Source: CAD feature listing. Evaluate the final solid. Frame: model axes, mm. Give positions to 0.01 mm unless a question says otherwise; leave off trailing zeros. Order: outer loops, then holes, each group sorted by start corner. A loop starts at its lowest first (then second) coordinate and runs counter-clockwise, first axis right, second up.
1) Material intervals for line 1 (Y direction, x = 17.5, z = 1); line 2 (Y direction, x = 7.5, z = 18), sorted ascending.
2) First-contact query: P1, Ø1.8, axis at y = -407.5, z = 10.5, coming from the -X side; P2, Ø12, axis at x = 6.5, z = 17.5, coming from the -Y side; P3, Ø8, axis at y = 407.793, z = 10, coming from the -X side; P4, Ø3.5, axis at y = -407.793, z = 10, coming from the +X side. Flat tips, straight axial feed; report the tip coordinate or a pass-through.
3) Section B-B, the plane x = 7.75. Return loops of the section in (y, z), plus the area to 3 significant figures.
```python
from build123d import *

# Parameters (mm, degrees)
F0_W     = 20
F0_H     = 20
F1_DEPTH = 417.793
F2_SIZE2 = 19.99999
F2_SIZE  = 19.99999
F3_SIZE  = 19.99999
F4_R     = 3
F5_DEPTH = 4
F6_R     = 3
F7_DEPTH = 4


# Not quite as in the source:
# - a fillet or chamfer is up to 0.001 mm smaller than in the source, because OpenCascade refuses the exact size


with BuildPart() as f1:
    # F0 (on Front) → F1 (new body, symmetric)
    with BuildSketch(Plane.XZ):
        with Locations((10, 10)):
            Rectangle(F0_W, F0_H)
    extrude(amount=F1_DEPTH, both=True)

    # F2 (size 20 and 20 in the source; OpenCascade refuses exactly that, so slightly less here)
    f2_edges = [f1.edges().sort_by_distance(p)[0] for p in [
        (20, -417.793, 10),
    ]]
    chamfer(f2_edges, length=F2_SIZE, length2=F2_SIZE2)

    # F3 (size 20 in the source; OpenCascade refuses exactly that, so slightly less here)
    f3_edges = [f1.edges().sort_by_distance(p)[0] for p in [
        (20, 417.793, 10),
    ]]
    chamfer(f3_edges, length=F3_SIZE)

    # F4 (on face) → F5 (cut)
    with BuildSketch(Plane(origin=(0, 0, 0), x_dir=(0, -1, 0), z_dir=(-1, 0, 0))):
        with Locations((-407.793, 10)):
            Circle(F4_R)
    extrude(amount=-F5_DEPTH, mode=Mode.SUBTRACT)

    # F6 (on face) → F7 (cut)
    with BuildSketch(Plane(origin=(0, 0, 0), x_dir=(0, -1, 0), z_dir=(-1, 0, 0))):
        with Locations((407.793, 10)):
            Circle(F6_R)
    extrude(amount=-F7_DEPTH, mode=Mode.SUBTRACT)


solid = f1.part
```
From the geometry:
1. line 1: y = -400.29 to 400.29
1. line 2: y = -410.29 to 410.29
2. P1: stops at x = 4
2. P2: stops at y = -417.29
2. P3: stops at x = 0
2. P4: stops at x = 11.75
3. outline: (-410.04, 0) - (410.04, 0) - (410.04, 20) - (-410.04, 20) - close
3. area: 16,400 mm2
